from build123d import *

# Parameters (mm, degrees)
BOSS_EXTRUDE1_DEPTH = 2.5


with BuildPart() as part:
    # Sketch1 → Boss-Extrude1 (new, symmetric)
    with BuildSketch(Plane.XY):
        Polygon((833.545659386, -88.691167375), (833.545659386, -73.941167375), (878.295659386, -73.941167375), (878.295659386, -84.191167375), (883.795659386, -84.191167375), (883.795659386, -73.941167375), (923.295659386, -73.941167375), (923.295659386, -84.191167375), (928.795659386, -84.191167375), (928.795659386, -73.941167375), (973.545659386, -73.941167375), (973.545659386, -88.691167375), (963.295659386, -88.691167375), (963.295659386, -94.191167375), (973.545659386, -94.191167375), (973.545659386, -141.191167375), (963.295659386, -141.191167375), (963.295659386, -146.691167375), (973.545659386, -146.691167375), (973.545659386, -193.691167375), (963.295659386, -193.691167375), (963.295659386, -199.191167375), (973.545659386, -199.191167375), (973.545659386, -213.941167375), (928.795659386, -213.941167375), (928.795659386, -203.691167375), (923.295659386, -203.691167375), (923.295659386, -213.941167375), (883.795659386, -213.941167375), (883.795659386, -203.691167375), (878.295659386, -203.691167375), (878.295659386, -213.941167375), (833.545659386, -213.941167375), (833.545659386, -199.191167375), (843.795659386, -199.191167375), (843.795659386, -193.691167375), (833.545659386, -193.691167375), (833.545659386, -146.691167375), (843.795659386, -146.691167375), (843.795659386, -141.191167375), (833.545659386, -141.191167375), (833.545659386, -94.191167375), (843.795659386, -94.191167375), (843.795659386, -88.691167375), align=None)
        Polygon((893.295659386, -88.691167375), (893.295659386, -93.941167375), (853.545659386, -93.941167375), (853.545659386, -107.441167375), (848.295659386, -107.441167375), (848.295659386, -127.941167375), (853.545659386, -127.941167375), (853.545659386, -159.94119829), (848.295659386, -159.941167375), (848.295659386, -180.441167375), (853.545659386, -180.441167375), (853.545659386, -193.941167375), (893.295659386, -193.941167375), (893.295659386, -199.191167375), (913.795659386, -199.191167375), (913.795659386, -193.941167375), (953.545659386, -193.941167375), (953.545659386, -180.441167375), (958.795659386, -180.441167375), (958.795659386, -159.941167375), (953.545659386, -159.94119829), (953.545659386, -127.941167375), (958.795659386, -127.941167375), (958.795659386, -107.441167375), (953.545659386, -107.441167375), (953.545659386, -93.941167375), (913.795659386, -93.941167375), (913.795659386, -88.691167375), align=None, mode=Mode.SUBTRACT)
    extrude(amount=BOSS_EXTRUDE1_DEPTH, both=True)


solid = part.part
Geometry check sheet. Reference: the model listing, model coordinates, mm. A direction names the side the tool comes from. Give positions to 0.01 mm unless a question says otherwise; leave off trailing zeros. Loops run counter-clockwise (first coordinate to the right, second up) from the corner with the lowest first, then second, coordinate; pieces in that order, holes last. Notation, with made-up numbers: (40.5, 77) -> (86.5, 77) arc R16 cw to (86.5, 82) -> close; hole circle Ø4 at (-27.5, 85.5). An arc over 180 degrees is marked (long way). Answer in a Markdown table with one row per item. Add a question column.
1) Draft check along Y on faces 1 (the face through (951, -213.941, 0)), 2 (the face through (973.546, -170, 0)), 3 (the face through (851, -180.441, 0)). Enter one of: pulls with the +Y half, pulls with the -Y half, needs draft (parallel to the pull), parting line crosses it, or undercut.
2) Cross-section at A-A on y = -178. Record the boundary of the cut face in (x, z), and give its area (4 significant figures).
3) Material ranges on probe 1 along Y at (x, z) = (955.5, -1.7); probe 2 along X at (y, z) = (-207, 0.6); probe 3 along Y at (x, z) = (968, -0.75), recorded low to high. Write a range as from..to.
4) Gauge pin test, flat ends, axial feed: P1, Ø1.5, axis at y = -92, z = -1, coming from the -X side; P2, Ø12, axis at x = 909, y = -183, coming from the -Z side (3 decimals); P3, Ø2.5, axis at y = -196, z = 1, coming from the +X side. Record the tip position at first contact, or that the pin passes through.
5) Cross-section at B-B on x = 861. Record the boundary of the cut face in (y, z).
6) Set-up check for faces 4 (the face through (883.796, -79, 0)), 5 (the face through (926, -203.691, 0)), 6 (the face through (904, -88.691, 0)), 7 (the face through (839, -146.691, 0)), 8 (the face through (963.296, -144, 0)): record each of +Z, -Z, +X, -X, +Y, -Y from which the full face is reachable in a straight line by a thin tool's end or side.
Outcome:
| question | item | result |
|---|---|---|
| 1 | face 1 | pulls with the -Y half |
| 1 | face 2 | needs draft |
| 1 | face 3 | undercut |
| 2 | outline | (833.55, -2.5) -> (848.3, -2.5) -> (848.3, 2.5) -> (833.55, 2.5) -> close; (958.8, -2.5) -> (973.55, -2.5) -> (973.55, 2.5) -> (958.8, 2.5) -> close |
| 2 | area | 147.5 mm^2 |
| 3 | probe 1 | y = -213.94..-180.44, -159.94..-127.94, -107.44..-73.94 |
| 3 | probe 2 | x = 833.55..878.3, 883.8..923.3, 928.8..973.55 |
| 3 | probe 3 | y = -213.94..-199.19, -193.69..-146.69, -141.19..-94.19, -88.69..-73.94 |
| 4 | P1 | stops at x = 843.8 |
| 4 | P2 | passes through |
| 4 | P3 | stops at x = 963.3 |
| 5 | outline | (-213.94, -2.5) -> (-193.94, -2.5) -> (-193.94, 2.5) -> (-213.94, 2.5) -> close; (-93.94, -2.5) -> (-73.94, -2.5) -> (-73.94, 2.5) -> (-93.94, 2.5) -> close |
| 6 | face 4 | +Z, -Z, +Y |
| 6 | face 5 | +Z, -Z, -Y |
| 6 | face 6 | +Z, -Z |
| 6 | face 7 | +Z, -Z, -X |
| 6 | face 8 | +Z, -Z, +X |
